Autodesk Inventor part; units mm, degrees
ref_plane "YZ Plane" through (0, 0, 0) normal (1, 0, 0) x (0, 1, 0)
ref_plane "XZ Plane" through (0, 0, 0) normal (0, 1, 0) x (-1, 0, 0)
ref_plane "XY Plane" through (0, 0, 0) normal (0, 0, 1) x (1, 0, 0)
sketch "Sketch1" plane through (0, 0, 0) normal (0, 0, 1) x (1, 0, 0)
  line L0 (0, 0) -> (64.8574, 0) construction
  line L1 (-60, -110) -> (60, -110)
  line L2 (60, -110) -> (60, 110)
  line L3 (60, 110) -> (-60, 110)
  line L4 (-60, 110) -> (-60, -110)
  line L5 (-60, -110) -> (60, 110) construction
  line L6 (60, -110) -> (-60, 110) construction
  dimension "d0" = 120
  dimension "d1" = 220
extrude "Extrusion1" add sketch "Sketch1" along normal blind 3
fillet "Fillet1" radius 10.25 4 edges at (60, 110, 1.5) (-60, 110, 1.5) (60, -110, 1.5) (-60, -110, 1.5)
sketch "Sketch2" plane through (0, 0, 3) normal (0, 0, 1) x (1, 0, 0)
  line L0 (0, 0) -> (47.0336, 0) construction
  line L1 (-30, -55) -> (30, -55)
  line L2 (30, -55) -> (30, 55)
  line L3 (30, 55) -> (-30, 55)
  line L4 (-30, 55) -> (-30, -55)
  line L5 (-30, -55) -> (30, 55) construction
  line L6 (30, -55) -> (-30, 55) construction
  line L7 (-57, 107) -> (57, 107)
  line L8 (57, 107) -> (57, -107)
  line L9 (57, -107) -> (-57, -107)
  line L10 (-57, -107) -> (-57, 107)
  dimension "d5" = 60
  dimension "d6" = 110
  dimension "d7" = -52
extrude "Extrusion2" add sketch "Sketch2" along normal blind 2 contours L4 L3 L2 L1 | L7 L8 L9 L10
fillet "Fillet2" radius 10.25 4 edges at (57, 107, 4) (-57, 107, 4) (-57, -107, 4) (57, -107, 4)
sketch "Sketch3" plane through (0, 0, 0) normal (0, 0, -1) x (-1, 0, 0)
  line L0 (18, 43.8265) -> (-18, 43.8265) construction
  line L1 (18, 46.8265) -> (-18, 46.8265)
  line L2 (-18, 40.8265) -> (18, 40.8265)
  arc A0 (18, 40.8265) -> (18, 46.8265) centre (18, 43.8265) ccw
  arc A1 (-18, 46.8265) -> (-18, 40.8265) centre (-18, 43.8265) ccw
  line L3 (-18, 49.8265) -> (18, 49.8265)
  arc A2 (18, 37.8265) -> (18, 49.8265) centre (18, 43.8265) ccw
  line L4 (18, 37.8265) -> (-18, 37.8265)
  arc A3 (-18, 49.8265) -> (-18, 37.8265) centre (-18, 43.8265) ccw
  point P0 (0, 0)
  point P1 (0, 43.8265)
  dimension "d11" = 18
  dimension "d12" = 6
  dimension "d15" = 3
extrude "Extrusion3" cut sketch "Sketch3" against normal through all contours A0 L2 A1 L1 | L3 A2 L4 A3
sketch "Sketch4" plane through (0, 0, 4) normal (0, 0, -1) x (-1, 0, 0)
  point P0 (0, 0)
properties part number "BackPlate"
Read the model definition and answer for the solid it produces. Units are mm, in the model's axes. A direction names the side the tool comes from. Coordinates: 2 decimals unless noted, no trailing zeros. Loops run counter-clockwise (first coordinate to the right, second up) from the corner with the lowest first, then second, coordinate; pieces in that order, holes last. Notation, with made-up numbers: (32.25, -8) - (81.25, -8) arc R17 cw to (81.25, 21) - close; hole circle Ø3 at (68.5, 17). An arc over 180 degrees is marked (long way). Answer in a Markdown table with one row per item.
1. Given pin 1 (1 mm diameter, centred on x = -24.5, z = 4, fed in from +Y), flat-ended and moving along its own axis, determine where the tip first touches the part or whether it passes through.
Conclusion:
| item | result |
|---|---|
| pin 1 | stops at y = 107 |
2. Find section D-D, the plane x = 21. Write down the section's boundary in (y, z), then the cut area to 3 significant figures.
Conclusion:
| item | result |
|---|---|
| outline | (-110, 0) - (38.63, 0) - (38.63, 5) - (-107, 5) - (-107, 3) - (-110, 3) - close; (49.02, 0) - (110, 0) - (110, 3) - (107, 3) - (107, 5) - (49.02, 5) - close |
| area | 1,040 mm² |
3. Find section A-A, the plane z = 4.15. Write down the section's boundary in (x, y).
Conclusion:
| item | result |
|---|---|
| outline | (-57, -96.75) arc R10.25 ccw to (-46.75, -107) - (46.75, -107) arc R10.25 ccw to (57, -96.75) - (57, 96.75) arc R10.25 ccw to (46.75, 107) - (-46.75, 107) arc R10.25 ccw to (-57, 96.75) - close; hole (-18, 37.83) - (18, 37.83) arc R6 ccw to (18, 49.83) - (-18, 49.83) arc R6 ccw to start |
4. Find section C-C, the plane x = -7.5. Write down the section's boundary in (y, z).
Conclusion:
| item | result |
|---|---|
| outline | (-110, 0) - (37.83, 0) - (37.83, 5) - (-107, 5) - (-107, 3) - (-110, 3) - close; (49.83, 0) - (110, 0) - (110, 3) - (107, 3) - (107, 5) - (49.83, 5) - close |
5. Find section B-B, the plane y = -51.5. Write down the section's boundary in (x, z).
Conclusion:
| item | result |
|---|---|
| outline | (-60, 0) - (60, 0) - (60, 3) - (57, 3) - (57, 5) - (-57, 5) - (-57, 3) - (-60, 3) - close |
6. Which of the six approach directions +Z, -Z, +X, -X, +Y, -Y give full straight-line access (tool end or side, diameter ignored) to faces 1 (the face through (-53.918, -104.077, 3.986)), 2 (the face through (-54.077, 103.918, 3.986)), 3 (the face through (54.077, -103.918, 3.986)), 4 (the face through (0, 37.826, 2))?
Conclusion:
| item | result |
|---|---|
| face 1 | +Z, -X, -Y |
| face 2 | +Z, -X, +Y |
| face 3 | +Z, +X, -Y |
| face 4 | +Z, -Z |
7. Straight lines are drawn through the part: line 1 (Y direction, x = 18.5, z = 1.8); line 2 (Y direction, x = -6, z = 3.9); line 3 (X direction, y = -1.5, z = 4.55). For each, find the intervals that lie inside material, in ascending order.
Conclusion:
| item | result |
|---|---|
| line 1 | y = -110 to 37.85, 49.81 to 110 |
| line 2 | y = -107 to 37.83, 49.83 to 107 |
| line 3 | x = -57 to 57 |
8. Determine the mould class of faces 5 (the face through (-56.918, 107.077, 1.521)), 6 (the face through (-1, 2, 0)), 7 (the face through (-24, 43.7, 2.5)), 8 (the face through (0, 49.826, 2)) for opening direction X: +X half, -X half, draft (parallel to the pull), parting line (faces both ways), or undercut.
Conclusion:
| item | result |
|---|---|
| face 5 | -X half |
| face 6 | draft |
| face 7 | undercut |
| face 8 | undercut |
